Could you check a few things on this model? Use its own coordinates, in mm. Give positions to 0.01 mm unless a question says otherwise; leave off trailing zeros. Order: outer loops, then holes, each group sorted by start corner. A loop starts at its lowest first (then second) coordinate and runs counter-clockwise, first axis right, second up. Notation, with made-up numbers: (81.25, 34.5) -> (93.25, 34.5) arc R29 ccw to (93.25, 64.5) -> close; hole circle Ø11 at (61.25, -39). An arc over 180 degrees is marked (long way). One line per item, written item: value.
```python
from build123d import *

# Parameters (mm, degrees)
F0_W        = 101.0252870619
F0_H        = 77.9844336212
F0_R        = 9.0586238997
F0_R_2      = 15.4013236799
F0_R_3      = 10.4395473454
F1_DEPTH    = 101.6
F2_T1_DEPTH = 132.7752870619
F2_T3_DEPTH = 109.7344336212


# Not quite as in the source:
# - a fillet or chamfer that OpenCascade refuses, or shapes differently, is made with other operations: its cross-section is extruded or revolved along the edge and cut away or added
# - a feature of the source that left no trace in its solid (it failed there, or was rolled back) is left out


with BuildPart() as f1:
    # F0 (on Front) → F1 (new body)
    with BuildSketch(Plane.XZ):
        with Locations((-15.3183694929, 6.5831001848)):
            Rectangle(F0_W, F0_H)
        with Locations((-11.3938301802, -10.6342416257)):
            Circle(F0_R, mode=Mode.SUBTRACT)
        with Locations((-30.6367408484, 20.7620896399)):
            Circle(F0_R_2, mode=Mode.SUBTRACT)
        with Locations((7.8490832821, 26.3324063271)):
            Circle(F0_R_3, mode=Mode.SUBTRACT)
    extrude(amount=F1_DEPTH)

    # F2: fillet of radius 6.35 on 7 edges, made by hand

    # F2_s2 → F2_t1 (cut)
    with BuildSketch(Plane.YZ.offset(-81.7060130239)):
        with BuildLine():
            ThreePointArc((-95.25, 45.5753169954), (-99.7401280605, 43.7154450559), (-101.6, 39.2253169954))
            Line((-101.6, 39.2253169954), (-101.6, 45.5753169954))
            Line((-101.6, 45.5753169954), (-95.25, 45.5753169954))
        make_face()
        with BuildLine():
            ThreePointArc((-95.25, -32.4091166258), (-99.7401280605, -30.5492446863), (-101.6, -26.0591166258))
            Line((-101.6, -26.0591166258), (-101.6, -32.4091166258))
            Line((-101.6, -32.4091166258), (-95.25, -32.4091166258))
        make_face()
    extrude(amount=F2_T1_DEPTH, mode=Mode.SUBTRACT)

    # F2_s4 → F2_t3 (cut)
    with BuildSketch(Plane.XY.offset(-48.2841166258)):
        with BuildLine():
            ThreePointArc((-65.8310130239, -95.25), (-63.9711410844, -99.7401280605), (-59.4810130239, -101.6))
            Line((-59.4810130239, -101.6), (-65.8310130239, -101.6))
            Line((-65.8310130239, -101.6), (-65.8310130239, -95.25))
        make_face()
        with BuildLine():
            ThreePointArc((35.1942740381, -95.25), (33.3344020986, -99.7401280605), (28.8442740381, -101.6))
            Line((28.8442740381, -101.6), (35.1942740381, -101.6))
            Line((35.1942740381, -101.6), (35.1942740381, -95.25))
        make_face()
    extrude(amount=F2_T3_DEPTH, mode=Mode.SUBTRACT)

    # F2_s5 → F2_t6 (revolve, cut)
    with BuildSketch(Plane.XY.offset(-10.6342416257)):
        with BuildLine():
            ThreePointArc((-2.3352062804, -95.25), (-0.475334341, -99.7401280605), (4.0147937196, -101.6))
            Line((4.0147937196, -101.6), (-2.3352062804, -101.6))
            Line((-2.3352062804, -101.6), (-2.3352062804, -95.25))
        make_face()
    revolve(axis=Axis((-11.3938301802, -101.6, -10.6342416257), (0, -1, 0)), mode=Mode.SUBTRACT)

    # F2_s7 → F2_t8 (revolve, cut)
    with BuildSketch(Plane.XY.offset(20.7620896399)):
        with BuildLine():
            ThreePointArc((-15.2354171685, -95.25), (-13.375545229, -99.7401280605), (-8.8854171685, -101.6))
            Line((-8.8854171685, -101.6), (-15.2354171685, -101.6))
            Line((-15.2354171685, -101.6), (-15.2354171685, -95.25))
        make_face()
    revolve(axis=Axis((-30.6367408484, -101.6, 20.7620896399), (0, -1, 0)), mode=Mode.SUBTRACT)

    # F2_s9 → F2_t10 (revolve, cut)
    with BuildSketch(Plane.XY.offset(26.3324063271)):
        with BuildLine():
            ThreePointArc((18.2886306275, -95.25), (20.1485025669, -99.7401280605), (24.6386306275, -101.6))
            Line((24.6386306275, -101.6), (18.2886306275, -101.6))
            Line((18.2886306275, -101.6), (18.2886306275, -95.25))
        make_face()
    revolve(axis=Axis((7.8490832821, -101.6, 26.3324063271), (0, -1, 0)), mode=Mode.SUBTRACT)


solid = f1.part
```
1) If I drill on line 1 along Z through (x, y) = (-31, -23); line 2 along X through (y, z) = (-29.5, -11); line 3 along Z through (x, y) = (-18.5, -67.5), over which ranges is the centre line in solid material (lowest first)?
Answer below:
line 1: z = -32.41 to 5.37, 36.16 to 45.58
line 2: x = -65.83 to -20.45, -2.34 to 35.19
line 3: z = -32.41 to -16.25, -5.02 to 11.28, 30.24 to 45.58
2) For P1, Ø11, axis at x = -11.39, z = -10.63, coming from the -Y side; P2, Ø24, axis at x = 7.85, z = 26.33, coming from the -Y side, each with a flat end and sliding along its axis, tell me the tip position at first contact or that it passes through.
Answer below:
P1: passes through
P2: stops at y = -99.42
3) Suppose I cut it at B-B, the plane z = 28. State how many separate pieces and enclosed holes the cut face has, then the cut area to 3 significant figures.
Answer below:
separate pieces: 3
enclosed holes: 0
area: 5,350 mm2
4) Suppose I cut it at A-A, the plane y = -89. Write out the boundary of the cut face in (x, z).
Answer below:
outline: (-65.83, -32.41) -> (35.19, -32.41) -> (35.19, 45.58) -> (-65.83, 45.58) -> close; hole circle Ø30.8 at (-30.64, 20.76); hole circle Ø18.12 at (-11.39, -10.63); hole circle Ø20.88 at (7.85, 26.33)
5) We'd pull the mould along X, two halves only. Please class faces 1 (the cylindrical face through (5.59, -46.96, 16.14)), 2 (the flat face through (-16, -47, 45.575)), 3 (the cylindrical face through (33.384, -99.69, 6.037)): +X half, -X half, draft (parallel to the pull), parting line (faces both ways), or undercut.
Answer below:
face 1: undercut
face 2: draft
face 3: +X half
